Verification items for the finished model (mm, model axes). Coordinates: 2 decimals unless noted, no trailing zeros. Write each loop counter-clockwise with the first axis right and the second up, starting at its lowest first coordinate (ties: lowest second). Pieces come first, ordered by that corner, then holes.
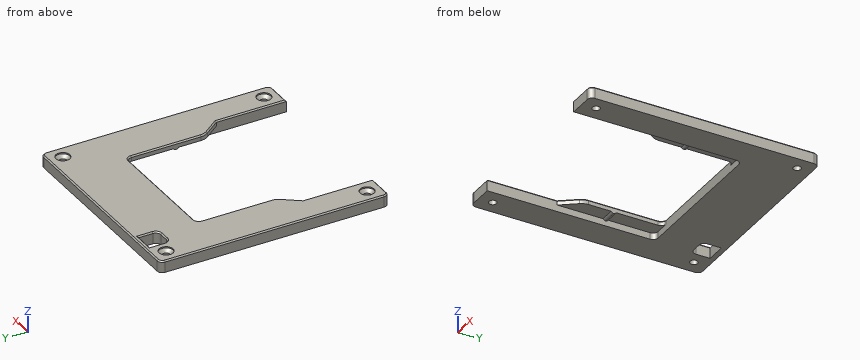
```python
from build123d import *

# Parameters (mm, degrees)
F1_DEPTH      = 2
F3_DEPTH      = 2.2
F5_DEPTH      = 25
F6_R          = 1.5
F7_DEPTH      = 4.2
F8_R          = 2.75
F9_DEPTH      = 2
F10_S5_R      = 1.5
F10_T6_DEPTH  = 5
F10_S11_R     = 1.5
F10_T12_DEPTH = 5
F10_S17_R     = 1.5
F10_T18_DEPTH = 5
F10_S23_R     = 1.5
F10_T24_DEPTH = 5
F11_W         = 5.6
F11_H         = 2
F12_DEPTH     = 0.6
F13_T1_DEPTH  = 8.4722813233
F13_T3_DEPTH  = 8.4722813233
F14_SIZE      = 0.5
F15_DEPTH     = 0.4


# Not quite as in the source:
# - a fillet or chamfer that OpenCascade refuses, or shapes differently, is made with other operations: its cross-section is extruded or revolved along the edge and cut away or added


with BuildPart() as f1:
    # F0 (on Top) → F1 (new body)
    with BuildSketch(Plane.XY):
        with BuildLine():
            Line((80, 0), (2, 0))
            ThreePointArc((2, 0), (0.5857864376, -0.5857864376), (0, -2))
            Line((0, -2), (0, -88))
            ThreePointArc((0, -88), (0.5857864376, -89.4142135624), (2, -90))
            Line((2, -90), (11.25, -90))
            Line((11.25, -90), (11.25, -62.5))
            Line((11.25, -62.5), (15.8564011104, -56.3307127986))
            ThreePointArc((15.8564011104, -56.3307127986), (16.5951030311, -54.9153368199), (16.85, -53.3392666362))
            Line((16.85, -53.3392666362), (16.85, -26))
            ThreePointArc((16.85, -26), (17.4357864376, -24.5857864376), (18.85, -24))
            Line((18.85, -24), (63.15, -24))
            ThreePointArc((63.15, -24), (64.5642135624, -24.5857864376), (65.15, -26))
            Line((65.15, -26), (65.15, -53.3392666362))
            ThreePointArc((65.15, -53.3392666362), (65.4048969689, -54.9153368199), (66.1435988896, -56.3307127986))
            Line((66.1435988896, -56.3307127986), (70.75, -62.5))
            Line((70.75, -62.5), (70.75, -90))
            Line((70.75, -90), (80, -90))
            ThreePointArc((80, -90), (81.4142135624, -89.4142135624), (82, -88))
            Line((82, -88), (82, -2))
            ThreePointArc((82, -2), (81.4142135624, -0.5857864376), (80, 0))
        make_face()
    extrude(amount=F1_DEPTH)

    # F2 (on face) → F3 (join)
    with BuildSketch(Plane(origin=(0, 0, 0), x_dir=(1, 0, 0), z_dir=(0, 0, -1))):
        with BuildLine():
            ThreePointArc((80, 0), (81.4142135624, 0.5857864376), (82, 2))
            Line((82, 2), (82, 88))
            ThreePointArc((82, 88), (81.4142135624, 89.4142135624), (80, 90))
            Line((80, 90), (70.75, 90))
            Line((70.75, 90), (70.75, 62.5))
            Line((70.75, 62.5), (70.75, 26))
            ThreePointArc((70.75, 26), (70.1642135624, 24.5857864376), (68.75, 24))
            Line((68.75, 24), (65.15, 24))
            Line((65.15, 24), (16.85, 24))
            Line((16.85, 24), (13.25, 24))
            ThreePointArc((13.25, 24), (11.8357864376, 24.5857864376), (11.25, 26))
            Line((11.25, 26), (11.25, 62.5))
            Line((11.25, 62.5), (11.25, 90))
            Line((11.25, 90), (2, 90))
            ThreePointArc((2, 90), (0.5857864376, 89.4142135624), (0, 88))
            Line((0, 88), (0, 2))
            ThreePointArc((0, 2), (0.5857864376, 0.5857864376), (2, 0))
            Line((2, 0), (80, 0))
        make_face()
    extrude(amount=F3_DEPTH)

    # F4 (on face) → F5 (cut)
    with BuildSketch(Plane.XY.offset(2)):
        with BuildLine():
            Line((18.3, -2), (10.5, -2))
            Line((10.5, -2), (10.5, -7.6))
            ThreePointArc((10.5, -7.6), (11.0857864376, -9.0142135624), (12.5, -9.6))
            Line((12.5, -9.6), (16.3, -9.6))
            ThreePointArc((16.3, -9.6), (17.7142135624, -9.0142135624), (18.3, -7.6))
            Line((18.3, -7.6), (18.3, -2))
        make_face()
    extrude(amount=-F5_DEPTH, mode=Mode.SUBTRACT)

    # F6 (on face) → F7 (cut)
    with BuildSketch(Plane.XY.offset(2)):
        with Locations((5.5, -84.5)):
            Circle(F6_R)
        with Locations((76.5, -84.5)):
            Circle(F6_R)
        with Locations((5.5, -5.5)):
            Circle(F6_R)
        with Locations((76.5, -5.5)):
            Circle(F6_R)
    extrude(amount=-F7_DEPTH, mode=Mode.SUBTRACT)

    # F8 (on face) → F9 (cut)
    with BuildSketch(Plane.XY.offset(2)):
        with Locations((5.5, -5.5)):
            Circle(F8_R)
        with Locations((76.5, -5.5)):
            Circle(F8_R)
        with Locations((76.5, -84.5)):
            Circle(F8_R)
        with Locations((5.5, -84.5)):
            Circle(F8_R)
    extrude(amount=-F9_DEPTH, mode=Mode.SUBTRACT)

    # F10: chamfer of 1.5 on 4 edges, made by hand


with BuildPart() as f10_tool2:
    # F10_s3 → F10_t4 (revolve)
    with BuildSketch(Plane.XZ.offset(84.5)):
        Polygon((8.25, 1.5), (6.75, 0), (8.25, 0), align=None)
    revolve(axis=Axis((5.5, -84.5, 0), (0, 0, 1)))

    # F10_s5 → F10_t6 (cut, symmetric)
    with BuildSketch(Plane.XY.offset(0.7)):
        with Locations((5.5, -84.5)):
            Circle(F10_S5_R)
    extrude(amount=F10_T6_DEPTH, both=True, mode=Mode.SUBTRACT)


with BuildPart() as f1_1:
    add(f1.part)

    # F10_t1: union F10_tool2
    add(f10_tool2.part)


with BuildPart() as f10_tool8:
    # F10_s9 → F10_t10 (revolve)
    with BuildSketch(Plane.XZ.offset(84.5)):
        Polygon((79.25, 1.5), (77.75, 0), (79.25, 0), align=None)
    revolve(axis=Axis((76.5, -84.5, 0), (0, 0, 1)))

    # F10_s11 → F10_t12 (cut, symmetric)
    with BuildSketch(Plane.XY.offset(0.7)):
        with Locations((76.5, -84.5)):
            Circle(F10_S11_R)
    extrude(amount=F10_T12_DEPTH, both=True, mode=Mode.SUBTRACT)


with BuildPart() as f1_2:
    add(f1_1.part)

    # F10_t7: union F10_tool8
    add(f10_tool8.part)


with BuildPart() as f10_tool14:
    # F10_s15 → F10_t16 (revolve)
    with BuildSketch(Plane.XZ.offset(5.5)):
        Polygon((8.25, 1.5), (6.75, 0), (8.25, 0), align=None)
    revolve(axis=Axis((5.5, -5.5, 0), (0, 0, 1)))

    # F10_s17 → F10_t18 (cut, symmetric)
    with BuildSketch(Plane.XY.offset(0.7)):
        with Locations((5.5, -5.5)):
            Circle(F10_S17_R)
    extrude(amount=F10_T18_DEPTH, both=True, mode=Mode.SUBTRACT)


with BuildPart() as f1_3:
    add(f1_2.part)

    # F10_t13: union F10_tool14
    add(f10_tool14.part)


with BuildPart() as f10_tool20:
    # F10_s21 → F10_t22 (revolve)
    with BuildSketch(Plane.XZ.offset(5.5)):
        Polygon((79.25, 1.5), (77.75, 0), (79.25, 0), align=None)
    revolve(axis=Axis((76.5, -5.5, 0), (0, 0, 1)))

    # F10_s23 → F10_t24 (cut, symmetric)
    with BuildSketch(Plane.XY.offset(0.7)):
        with Locations((76.5, -5.5)):
            Circle(F10_S23_R)
    extrude(amount=F10_T24_DEPTH, both=True, mode=Mode.SUBTRACT)


with BuildPart() as f1_4:
    add(f1_3.part)

    # F10_t19: union F10_tool20
    add(f10_tool20.part)

    # F11 (on face) → F12 (join)
    with BuildSketch(Plane(origin=(0, 0, 0), x_dir=(1, 0, 0), z_dir=(0, 0, -1))):
        with Locations((14.05, 43.5)):
            Rectangle(F11_W, F11_H)
        with Locations((67.95, 43.5)):
            Rectangle(F11_W, F11_H)
    extrude(amount=F12_DEPTH)

    # F13: fillet of radius 1.4 on 4 edges, made by hand

    # F13_s2 → F13_t1 (cut)
    with BuildSketch(Plane.YZ.offset(11.25)):
        with BuildLine():
            ThreePointArc((-42.5, 0), (-43.0008384595, -0.4409673646), (-43.6489125293, -0.6))
            Line((-43.6489125293, -0.6), (-42.5, -0.6))
            Line((-42.5, -0.6), (-42.5, 0))
        make_face()
        with BuildLine():
            ThreePointArc((-43.3510874707, -0.6), (-43.9991615405, -0.4409673646), (-44.5, 0))
            Line((-44.5, 0), (-44.5, -0.6))
            Line((-44.5, -0.6), (-43.3510874707, -0.6))
        make_face()
    extrude(amount=F13_T1_DEPTH, mode=Mode.SUBTRACT)

    # F13_s4 → F13_t3 (cut)
    with BuildSketch(Plane.YZ.offset(62.2777186767)):
        with BuildLine():
            ThreePointArc((-43.6489125293, -0.6), (-43.0008384595, -0.4409673646), (-42.5, 0))
            Line((-42.5, 0), (-42.5, -0.6))
            Line((-42.5, -0.6), (-43.6489125293, -0.6))
        make_face()
        with BuildLine():
            ThreePointArc((-44.5, 0), (-43.9991615405, -0.4409673646), (-43.3510874707, -0.6))
            Line((-43.3510874707, -0.6), (-44.5, -0.6))
            Line((-44.5, -0.6), (-44.5, 0))
        make_face()
    extrude(amount=F13_T3_DEPTH, mode=Mode.SUBTRACT)

    # F14
    f14_edges = [f1_4.edges().sort_by_distance(p)[0] for p in [
        (0.585786, -0.585786, 2),
        (41, 0, 2),
        (0, -45, 2),
        (10.5, -4.8, 2),
        (14.4, -2, 2),
        (18.3, -4.8, 2),
        (17.714214, -9.014214, 2),
        (14.4, -9.6, 2),
        (11.085786, -9.014214, 2),
        (81.414214, -0.585786, 2),
        (82, -45, 2),
        (11.25, -76.25, 2),
        (6.625, -90, 2),
        (0.585786, -89.414214, 2),
        (81.414214, -89.414214, 2),
        (75.375, -90, 2),
        (70.75, -76.25, 2),
        (68.446799, -59.415356, 2),
        (65.404897, -54.915337, 2),
        (65.15, -39.669633, 2),
        (64.564214, -24.585786, 2),
        (41, -24, 2),
        (17.435786, -24.585786, 2),
        (16.85, -39.669633, 2),
        (16.595103, -54.915337, 2),
        (13.553201, -59.415356, 2),
    ]]
    chamfer(f14_edges, length=F14_SIZE)

    # F15 (add): a face of the model
    f15_faces = [f1_4.faces().sort_by_distance(p)[0] for p in [
        (80.5532838324, -1.4467161676, -2.2),
    ]]
    extrude(f15_faces, amount=F15_DEPTH)


solid = f1_4.part
```
1. Sectioned sample at B-B, the plane y = -70. Record the boundary of the cut face in (x, z).
2. Sectioned sample at D-D, the plane x = 49.5. Record the boundary of the cut face in (y, z).
3. Sectioned sample at C-C, the plane x = 5.5. Record the boundary of the cut face in (y, z).
4. Sectioned sample at A-A, the plane y = -84.5. Record the boundary of the cut face in (x, z).
5. Material ranges on L1, parallel to Y at x = 5.5, z = -1.15; L2, parallel to X at y = -68.5, z = 1.4; L3, parallel to X at y = -84.5, z = -1.5, recorded low to high.
6. Gauge pin test, flat ends, axial feed: P1, Ø2, axis at x = 28.5, z = -2, coming from the -Y side; P2, Ø8.5, axis at x = 66, y = -34, coming from the -Z side; P3, Ø2, axis at x = 68, z = 1, coming from the -Y side. Record the tip position at first contact, or that the pin passes through.
Outcome:
1. outline: (0, -2.6) - (11.25, -2.6) - (11.25, 1.5) - (10.75, 2) - (0.5, 2) - (0, 1.5) - close; (70.75, -2.6) - (82, -2.6) - (82, 1.5) - (81.5, 2) - (71.25, 2) - (70.75, 1.5) - close
2. outline: (-24, -2.6) - (0, -2.6) - (0, 1.5) - (-0.5, 2) - (-23.5, 2) - (-24, 1.5) - close
3. outline: (-90, -2.6) - (-86, -2.6) - (-86, 0.25) - (-87.25, 1.5) - (-87.25, 2) - (-89.5, 2) - (-90, 1.5) - close; (-83, -2.6) - (-7, -2.6) - (-7, 0.25) - (-8.25, 1.5) - (-8.25, 2) - (-81.75, 2) - (-81.75, 1.5) - (-83, 0.25) - close; (-4, -2.6) - (0, -2.6) - (0, 1.5) - (-0.5, 2) - (-2.75, 2) - (-2.75, 1.5) - (-4, 0.25) - close
4. outline: (0, -2.6) - (4, -2.6) - (4, 0.25) - (2.75, 1.5) - (2.75, 2) - (0.5, 2) - (0, 1.5) - close; (7, -2.6) - (11.25, -2.6) - (11.25, 1.5) - (10.75, 2) - (8.25, 2) - (8.25, 1.5) - (7, 0.25) - close; (70.75, -2.6) - (75, -2.6) - (75, 0.25) - (73.75, 1.5) - (73.75, 2) - (71.25, 2) - (70.75, 1.5) - close; (78, -2.6) - (82, -2.6) - (82, 1.5) - (81.5, 2) - (79.25, 2) - (79.25, 1.5) - (78, 0.25) - close
5. L1: y = -90 to -86, -83 to -7, -4 to 0
5. L2: x = 0 to 11.25, 70.75 to 82
5. L3: x = 0 to 4, 7 to 11.25, 70.75 to 75, 78 to 82
6. P1: stops at y = -24
6. P2: stops at z = 0
6. P3: stops at y = -60.16
